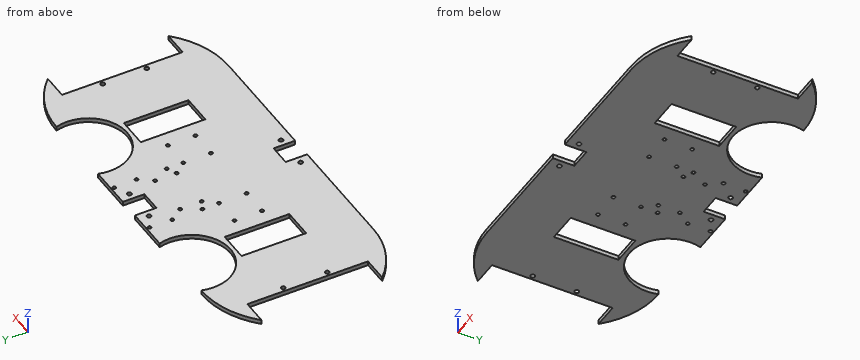
from build123d import *

# Parameters (mm, degrees)
SKETCH1_R           = 2
BOSS_EXTRUDE1_DEPTH = 5
SKETCH2_R           = 2.5
SKETCH2_W           = 35
SKETCH2_H           = 75
CUT_EXTRUDE1_DEPTH  = 10
SKETCH4_R           = 2
CUT_EXTRUDE3_DEPTH  = 10
SKETCH5_R           = 2.5
CUT_EXTRUDE4_DEPTH  = 10
SKETCH6_W           = 25
SKETCH6_H           = 25
CUT_EXTRUDE5_DEPTH  = 10


with BuildPart() as part:
    # Sketch1 → Boss-Extrude1 (new body)
    with BuildSketch(Plane.XY):
        with BuildLine():
            Line((77, 150.635083269), (106.477021815, 150.635083269))
            ThreePointArc((106.477021815, 150.635083269), (73.792570992, 172.830527842), (35.06273753, 180.635083269))
            ThreePointArc((35.06273753, 180.635083269), (-7.999345575, 122.571508006), (-51.06142868, 180.635083269))
            Line((-51.06142868, 180.635083269), (-178.81309626, 180.635083269))
            ThreePointArc((-178.81309626, 180.635083269), (-221.875179365, 122.571508006), (-264.93726247, 180.635083269))
            ThreePointArc((-264.93726247, 180.635083269), (-303.667095932, 172.830527842), (-336.351546756, 150.635083269))
            Line((-336.351546756, 150.635083269), (-306.874524941, 150.635083269))
            Line((-306.874524941, 150.635083269), (-306.874524941, 10.635083269))
            Line((-306.874524941, 10.635083269), (-336.351546756, 10.635083269))
            ThreePointArc((-336.351546756, 10.635083269), (-303.667095932, -11.560361304), (-264.93726247, -19.364916731))
            Line((-264.93726247, -19.364916731), (35.06273753, -19.364916731))
            ThreePointArc((35.06273753, -19.364916731), (73.792570992, -11.560361304), (106.477021815, 10.635083269))
            Line((106.477021815, 10.635083269), (77, 10.635083269))
            Line((77, 10.635083269), (77, 150.635083269))
        make_face()
        with Locations((-151.935, 116.015296492)):
            Circle(SKETCH1_R, mode=Mode.SUBTRACT)
        with Locations((-140.936318375, 110.635083269)):
            Circle(SKETCH1_R, mode=Mode.SUBTRACT)
        with Locations((-140.936318375, 135.635083269)):
            Circle(SKETCH1_R, mode=Mode.SUBTRACT)
        with Locations((-151.935, 151.015296492)):
            Circle(SKETCH1_R, mode=Mode.SUBTRACT)
        with Locations((-151.436318375, 177.135083269)):
            Circle(SKETCH1_R, mode=Mode.SUBTRACT)
        with Locations((-88.936318375, 110.635083269)):
            Circle(SKETCH1_R, mode=Mode.SUBTRACT)
        with Locations((-77.935, 116.015296492)):
            Circle(SKETCH1_R, mode=Mode.SUBTRACT)
        with Locations((-88.936318375, 135.635083269)):
            Circle(SKETCH1_R, mode=Mode.SUBTRACT)
        with Locations((-77.935, 151.015296492)):
            Circle(SKETCH1_R, mode=Mode.SUBTRACT)
        with Locations((-78.436318375, 177.135083269)):
            Circle(SKETCH1_R, mode=Mode.SUBTRACT)
    extrude(amount=-BOSS_EXTRUDE1_DEPTH)

    # Sketch2 → Cut-Extrude1 (cut)
    with BuildSketch(Plane(origin=(0, 0, -5), x_dir=(-1, 0, 0), z_dir=(0, 0, -1))):
        with Locations((301.874524941, 106.135083269)):
            Circle(SKETCH2_R)
        with Locations(Location((301.874524941, 55.135083269, 0), (0, 0, 180))):
            Circle(SKETCH2_R)
        with Locations((-72, 55.135083269)):
            Circle(SKETCH2_R)
        with Locations(Location((-72, 106.135083269, 0), (0, 0, 180))):
            Circle(SKETCH2_R)
        with Locations((219.374524941, 80.635083269)):
            Rectangle(SKETCH2_W, SKETCH2_H)
        with Locations((10.5, 80.635083269)):
            Rectangle(SKETCH2_W, SKETCH2_H)
    extrude(amount=-CUT_EXTRUDE1_DEPTH, mode=Mode.SUBTRACT)

    # Sketch4 → Cut-Extrude3 (cut)
    with BuildSketch(Plane(origin=(0, 0, -5), x_dir=(-1, 0, 0), z_dir=(0, 0, -1))):
        with Locations((46, 64.695083269)):
            Circle(SKETCH4_R)
        with Locations((46, 96.695083269)):
            Circle(SKETCH4_R)
        with Locations((78, 64.695083269)):
            Circle(SKETCH4_R)
        with Locations((78, 96.695083269)):
            Circle(SKETCH4_R)
        with Locations(Location((151.874524941, 64.695083269, 0), (0, 0, 180))):
            Circle(SKETCH4_R)
        with Locations(Location((183.874524941, 64.695083269, 0), (0, 0, 180))):
            Circle(SKETCH4_R)
        with Locations(Location((183.874524941, 96.695083269, 0), (0, 0, 180))):
            Circle(SKETCH4_R)
        with Locations(Location((151.874524941, 96.695083269, 0), (0, 0, 180))):
            Circle(SKETCH4_R)
    extrude(amount=-CUT_EXTRUDE3_DEPTH, mode=Mode.SUBTRACT)

    # Sketch5 → Cut-Extrude4 (cut)
    with BuildSketch(Plane(origin=(0, 0, -5), x_dir=(-1, 0, 0), z_dir=(0, 0, -1))):
        with Locations((94.63726247, 168.635083269)):
            Circle(SKETCH5_R)
        with Locations((135.23726247, 168.635083269)):
            Circle(SKETCH5_R)
        with Locations(Location((94.63726247, -7.364916731, 0), (0, 0, 180))):
            Circle(SKETCH5_R)
        with Locations(Location((135.23726247, -7.364916731, 0), (0, 0, 180))):
            Circle(SKETCH5_R)
    extrude(amount=-CUT_EXTRUDE4_DEPTH, mode=Mode.SUBTRACT)

    # Sketch6 → Cut-Extrude5 (cut)
    with BuildSketch(Plane(origin=(0, 0, -5), x_dir=(-1, 0, 0), z_dir=(0, 0, -1))):
        with Locations((114.939524941, -6.864916731)):
            Rectangle(SKETCH6_W, SKETCH6_H)
        with Locations((114.939524941, 168.135083269)):
            Rectangle(SKETCH6_W, SKETCH6_H)
    extrude(amount=-CUT_EXTRUDE5_DEPTH, mode=Mode.SUBTRACT)


solid = part.part
The listing builds one solid part. Answer for the finished solid, in the listing's coordinates (mm). Give positions to 0.01 mm unless a question says otherwise; leave off trailing zeros. Order: outer loops, then holes, each group sorted by start corner. A loop starts at its lowest first (then second) coordinate and runs counter-clockwise, first axis right, second up. Notation, with made-up numbers: (85.5, 37.25) - (132.5, 37.25) arc R22 ccw to (132.5, 47.25) - close; hole circle Ø3 at (-36, 65). An arc over 180 degrees is marked (long way). Use one line per item in the form item = value.
1) Find section B-B on y = 128. Determine the outline of the cut face in (x, z), and give its area (3 significant figures).
Verdict:
outline = (-306.87, -5) - (-243.3, -5) - (-243.3, 0) - (-306.87, 0) - close; (-200.45, -5) - (-29.43, -5) - (-29.43, 0) - (-200.45, 0) - close; (13.43, -5) - (77, -5) - (77, 0) - (13.43, 0) - close
area = 1,490 mm^2
2) Find section A-A on y = 48. Determine the outline of the cut face in (x, z).
Verdict:
outline = (-306.87, -5) - (-236.87, -5) - (-236.87, 0) - (-306.87, 0) - close; (-201.87, -5) - (-28, -5) - (-28, 0) - (-201.87, 0) - close; (7, -5) - (77, -5) - (77, 0) - (7, 0) - close
3) Each of these flat-tipped pins is pushed along its axis until it touches: pin 1 (1.5 mm diameter, centred on x = -320, z = -2, fed in from +Y); pin 2 (2.5 mm diameter, centred on x = -110, z = -2.5, fed in from -Y); pin 3 (2.5 mm diameter, centred on x = -316, z = -3.5, fed in from -Y). Where does it stop, or does it pass through?
Verdict:
pin_1 = 164.6
pin_2 = 5.64
pin_3 = -6.08
4) Find section C-C on x = -34. Determine the outline of the cut face in (y, z), and give its area (3 significant figures).
Verdict:
outline = (-19.36, -5) - (130.84, -5) - (130.84, 0) - (-19.36, 0) - close
area = 751 mm^2
5) Find section D-D on x = 29.5. Determine the outline of the cut face in (y, z).
Verdict:
outline = (-19.36, -5) - (142.7, -5) - (142.7, 0) - (-19.36, 0) - close
6) Consider probe 1 along X at (y, z) = (84.5, -0.65); probe 2 along X at (y, z) = (110, -0.9); probe 3 along X at (y, z) = (149.5, -1.95). Determine where each line is inside the solid, lowest interval first. Write a range as [from, to].
Verdict:
probe_1 = [-306.87, -236.87], [-201.87, -28], [7, 77]
probe_2 = [-306.87, -236.87], [-201.87, -142.83], [-139.04, -90.83], [-87.04, -28], [7, 77]
probe_3 = [-306.87, -263.09], [-180.66, -153.24], [-150.63, -79.24], [-76.63, -49.21], [33.21, 77]
